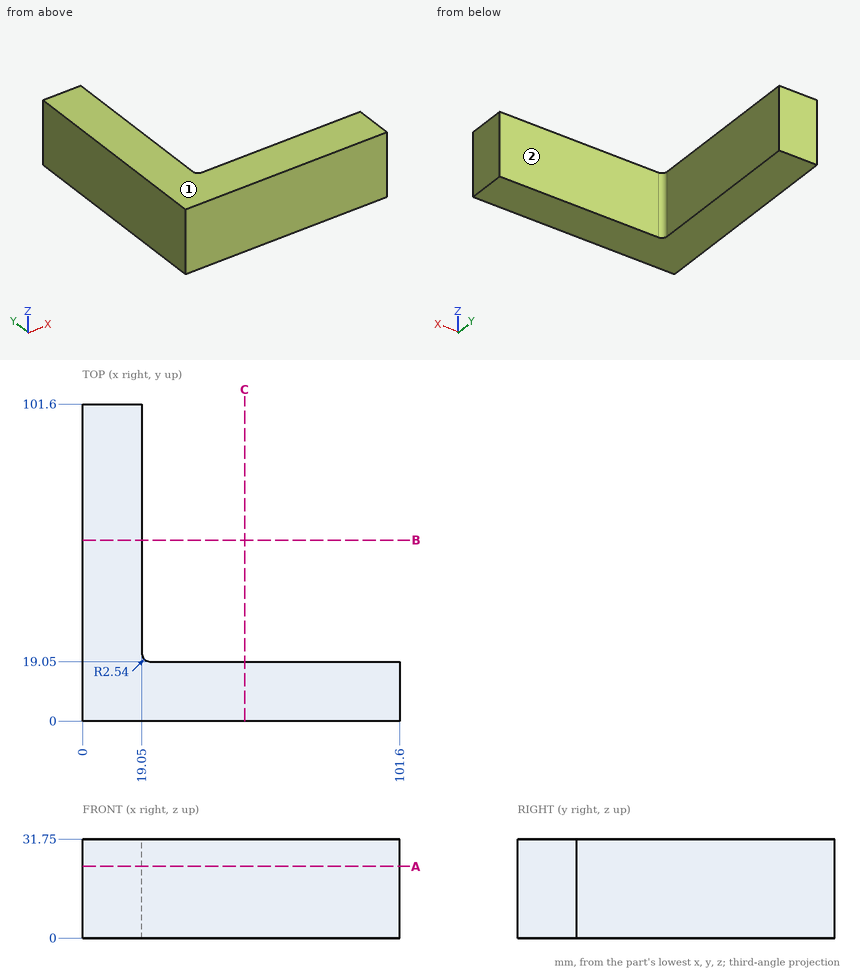
Can you work these out from the drawing? Everything is in mm from the part's minimum corner. A direction names the side the tool comes from. Give positions to 0.01 mm unless a question says otherwise; leave off trailing zeros. Order: outer loops, then holes, each group sorted by start corner. A loop starts at its lowest first (then second) coordinate and runs counter-clockwise, first axis right, second up. Notation, with made-up numbers: M 38,-8 L 53,-8 A18 cw 53,16 Z; hole C -9.75,-35.5 d10. An arc over 180 degrees is marked long. Write item = value, one per line. Start each with the question number.
Q1. For the marked faces 1 and 2, which set-ups out of +Z, -Z, +X, -X, +Y, -Y let a thin tool reach every point of the face, with its end or its side?
Q2. I need wall thicknesses on probe 1 along X at (y, z) = (90.5, 26); probe 2 along X at (y, z) = (20.5, 16). Which ranges of each line are inside material? Lowest first, please. Write a range as [from, to].
Q3. Suppose I cut it at B-B (y = 58). Write out the boundary of the cut face in (x, z), plus the area to 3 significant figures.
Q4. Will this pin go through, and if not, where does the flat tip stop? pin 1 Ø9.5 at (y, z) = (52, 16) entering from +X.
Q5. Suppose I cut it at A-A (z = 23). Write out the boundary of the cut face in (x, y), plus the area to 3 significant figures.
Check result:
q1.face_1 = +Z, +X, -X, +Y, -Y
q1.face_2 = +Z, -Z, +X, +Y
q2.probe_1 = [0, 19.05]
q2.probe_2 = [0, 19.3]
q3.outline = M 0,0 L 19.05,0 L 19.05,31.75 L 0,31.75 Z
q3.area = 605 mm2
q4.pin_1 = 19.05
q5.outline = M 0,0 L 101.6,0 L 101.6,19.05 L 21.59,19.05 A2.54 cw 19.05,21.59 L 19.05,101.6 L 0,101.6 Z
q5.area = 3,510 mm2
